Read the model definition and answer for the solid it produces. Units are mm, in the model's axes. A direction names the side the tool comes from. Give positions to 0.01 mm unless a question says otherwise; leave off trailing zeros. Loops run counter-clockwise (first coordinate to the right, second up) from the corner with the lowest first, then second, coordinate; pieces in that order, holes last. Notation, with made-up numbers: (37, 79.25) - (83, 79.25) arc R18 ccw to (83, 113.25) - close; hole circle Ø8 at (-31, 49). An arc over 180 degrees is marked (long way). Use a Markdown table: item, result. Add a question column.
Item 1: A cutting plane is placed at C-C (x = 3.25). Determine the outline of the cut face in (y, z).
Item 2: A cutting plane is placed at A-A (z = 0). Determine the outline of the cut face in (x, y), plus the area to 3 significant figures.
Item 3: Which of the six approach directions +Z, -Z, +X, -X, +Y, -Y give full straight-line access (tool end or side, diameter ignored) to faces 4 (the face through (-0.038, -43.953, -10.148)), 5 (the face through (-0.995, -45.701, -9.548))?
Item 4: Consider probe 1 along Y at (x, z) = (1.25, -14); probe 2 along Y at (x, z) = (2.5, -10); probe 3 along Y at (x, z) = (0.5, -7.5). Determine where each line is inside the solid, lowest interval first. Write a range as [from, to].
Item 5: A cutting plane is placed at B-B (x = 1.75). Determine the outline of the cut face in (y, z), plus the area to 3 significant figures.
Item 6: For a pull along Y with two mould halves and no side action, classify faces 1 (the face through (-0.051, -44.919, 7.114)), 2 (the face through (0.02, -46.545, -9.725)), 3 (the face through (0.99, -45.69, -9.55)) as +Y half, -Y half, draft (parallel to the pull), parting line (faces both ways), or undercut.
Item 7: Each of these flat-tipped pins is pushed along its axis until it touches: P1, Ø1.5, axis at x = -3, z = -3.5, coming from the +Y side; P2, Ø4, axis at x = 1.5, z = -21.5, coming from the +Y side. Where does it stop, or does it pass through?
from build123d import *

# Parameters (mm, degrees)
REVOLVE1_ANGLE           = 33
REVOLVE1_OTHER_WAY_ANGLE = 10
FILLET1_START            = -5
FILLET1_DEPTH            = 10


with BuildPart() as part:
    # Sketch1 → Revolve1 (revolve)
    with BuildSketch(Plane(origin=(0, 0, 0), x_dir=(1, 0, 0), z_dir=(0, 0, -1))):
        with BuildLine():
            Line((-3.640625, 46), (-1.217705098, 46))
            ThreePointArc((-1.217705098, 46), (-0.919977315, 46.165994111), (-0.904655581, 46.506524758))
            Line((-0.904655581, 46.506524758), (-1.426393202, 47.55))
            Line((-1.426393202, 47.55), (1.426393202, 47.55))
            Line((1.426393202, 47.55), (0.904655581, 46.506524758))
            ThreePointArc((0.904655581, 46.506524758), (0.919977315, 46.165994111), (1.217705098, 46))
            Line((1.217705098, 46), (3.640625, 46))
            ThreePointArc((3.640625, 46), (3.379766977, 45.370233023), (2.75, 45.109375))
            Line((2.75, 45.109375), (-2.75, 45.109375))
            ThreePointArc((-2.75, 45.109375), (-3.379766977, 45.370233023), (-3.640625, 46))
        make_face()
    revolve(axis=Axis((0, 0, 0), (1, 0, 0)), revolution_arc=REVOLVE1_ANGLE)

    # Sketch1 → Revolve1 other way (revolve)
    with BuildSketch(Plane(origin=(0, 0, 0), x_dir=(1, 0, 0), z_dir=(0, 0, -1))):
        with BuildLine():
            Line((-3.640625, 46), (-1.217705098, 46))
            ThreePointArc((-1.217705098, 46), (-0.919977315, 46.165994111), (-0.904655581, 46.506524758))
            Line((-0.904655581, 46.506524758), (-1.426393202, 47.55))
            Line((-1.426393202, 47.55), (1.426393202, 47.55))
            Line((1.426393202, 47.55), (0.904655581, 46.506524758))
            ThreePointArc((0.904655581, 46.506524758), (0.919977315, 46.165994111), (1.217705098, 46))
            Line((1.217705098, 46), (3.640625, 46))
            ThreePointArc((3.640625, 46), (3.379766977, 45.370233023), (2.75, 45.109375))
            Line((2.75, 45.109375), (-2.75, 45.109375))
            ThreePointArc((-2.75, 45.109375), (-3.379766977, 45.370233023), (-3.640625, 46))
        make_face()
    revolve(axis=Axis((0, 0, 0), (-1, 0, 0)), revolution_arc=REVOLVE1_OTHER_WAY_ANGLE)

    # Fillet1: read off the stored shape, not the designer's step
    # Fillet1 outline → Fillet1 (cut)
    with BuildSketch(Plane.YZ.offset(FILLET1_START)):
        with BuildLine():
            ThreePointArc((-46.351849466, 8.173081667), (-45.085567377, 7.385144883), (-44.716561853, 5.94010176))
            ThreePointArc((-44.716561853, 5.94010176), (-44.580361526, 6.888184024), (-44.424062234, 7.833160764))
            Line((-44.424062234, 7.833160764), (-46.351849466, 8.173081667))
        make_face()
    extrude(amount=FILLET1_DEPTH, mode=Mode.SUBTRACT)


solid = part.part
Geometry says:
| question | item | result |
|---|---|---|
| 1 | outline | (-45.35, 7.68) arc R46 ccw to (-38.58, -25.05) - (-37.96, -24.65) arc R45.26 cw to (-44.76, 6.71) arc R2 ccw to start |
| 2 | outline | (-3.64, -46) - (-1.22, -46) arc R0.35 cw to (-0.9, -46.51) - (-1.43, -47.55) - (1.43, -47.55) - (0.9, -46.51) arc R0.35 cw to (1.22, -46) - (3.64, -46) arc R0.89 ccw to (2.75, -45.11) - (-2.75, -45.11) arc R0.89 ccw to start |
| 2 | area | 9.51 mm² |
| 3 | face 4 | +X, -X, +Y |
| 3 | face 5 | -X |
| 4 | probe 1 | [-45.44, -45.07], [-43.82, -42.88] |
| 4 | probe 2 | [-44.9, -43.99] |
| 4 | probe 3 | [-46.95, -44.48] |
| 5 | outline | (-45.35, 7.68) arc R46 ccw to (-38.58, -25.05) - (-37.83, -24.57) arc R45.11 cw to (-44.72, 5.94) arc R2 ccw to start |
| 5 | area | 29.8 mm² |
| 6 | face 1 | +Y half |
| 6 | face 2 | -Y half |
| 6 | face 3 | undercut |
| 7 | P1 | y = -44.91 |
| 7 | P2 | y = -38.5 |
